Source: three-view drawing plus pictorial views. Frame: mm from the lowest corner of the part. A direction names the side the tool comes from. Coordinates: 2 decimals unless noted, no trailing zeros. Order: outer loops, then holes, each group sorted by start corner. A loop starts at its lowest first (then second) coordinate and runs counter-clockwise, first axis right, second up. Notation, with made-up numbers: (-13.75, -31.5) - (4.25, -31.5) arc R27 cw to (4.25, -8.5) - close; hole circle Ø9 at (-39, 49). An arc over 180 degrees is marked (long way). One line per question, with ' | ' between items.
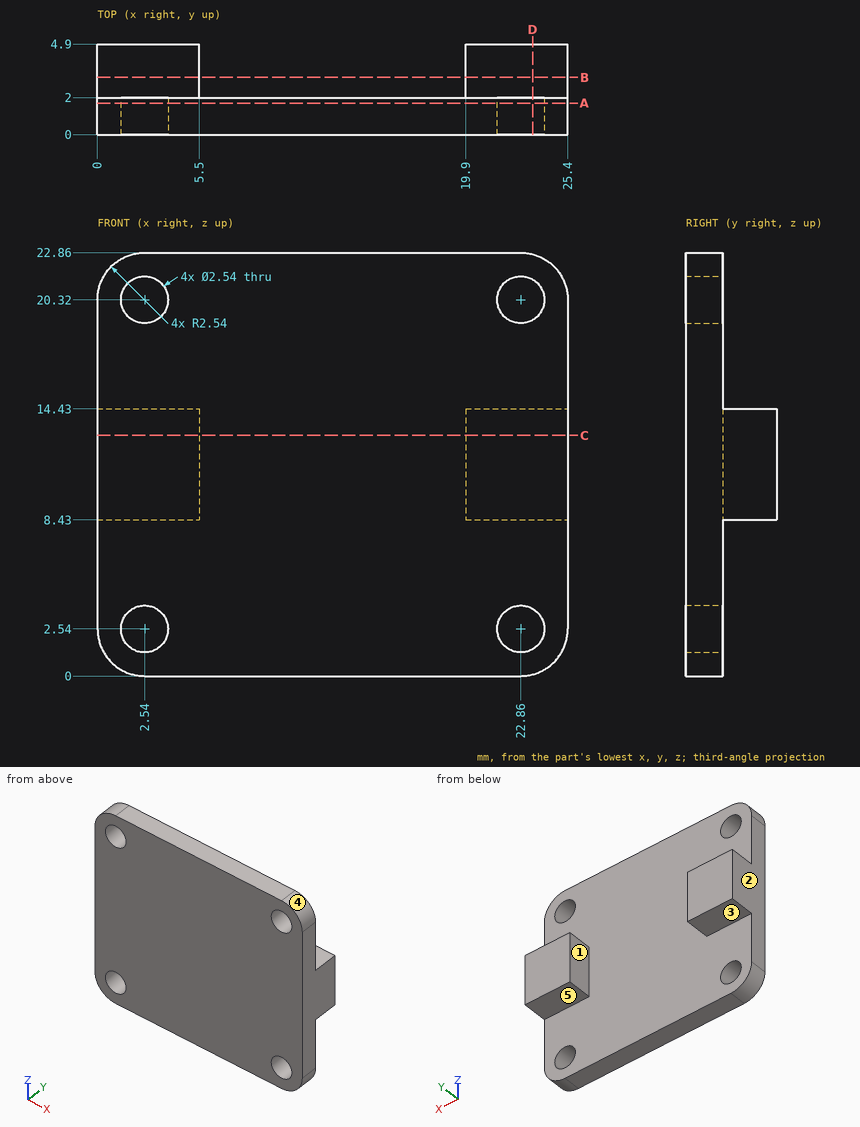
(1) Pin query (flat end, axial travel): P1, Ø10, axis at x = 7, z = 5.5, coming from the +Y side; P2, Ø3, axis at x = 2.54, z = 20.32, coming from the +Y side; P3, Ø1.5, axis at x = 23, y = 3.5, coming from the -Z side; P4, Ø1, axis at x = 13, y = 4, coming from the -Z side. Return the tip coordinate at first contact, or that it passes through.
Taken from the geometry:
P1: stops at y = 4.9 | P2: stops at y = 2 | P3: stops at z = 8.43 | P4: passes through
(2) Pull-direction query (X, two-part tool) for the marked faces 1, 2 and 3; classes: pulls with the +X half, pulls with the -X half, needs draft (parallel to the pull), parting line crosses it, or undercut.
Taken from the geometry:
face 1: undercut | face 2: pulls with the -X half | face 3: needs draft
(3) Cut plane C-C (z = 13). Return the cut outline in (x, y), and give its area (3 significant figures).
Taken from the geometry:
outline: (0, 0) - (25.4, 0) - (25.4, 4.9) - (19.9, 4.9) - (19.9, 2) - (5.5, 2) - (5.5, 4.9) - (0, 4.9) - close | area: 82.7 mm²
(4) Material intervals for L1, parallel to X at y = 1.05, z = 2.54; L2, parallel to Z at x = 2.54, y = 1.25; L3, parallel to Z at x = 1.75, y = 1.9, sorted ascending. Write a range as from..to.
Taken from the geometry:
L1: x = 0..1.27, 3.81..21.59, 24.13..25.4 | L2: z = 0..1.27, 3.81..19.05, 21.59..22.86 | L3: z = 0.13..1.55, 3.53..19.33, 21.31..22.73
(5) Cut plane A-A (y = 1.7). Return the cut outline in (x, z).
Taken from the geometry:
outline: (0, 2.54) arc R2.54 ccw to (2.54, 0) - (22.86, 0) arc R2.54 ccw to (25.4, 2.54) - (25.4, 20.32) arc R2.54 ccw to (22.86, 22.86) - (2.54, 22.86) arc R2.54 ccw to (0, 20.32) - close; hole circle Ø2.54 at (2.54, 2.54); hole circle Ø2.54 at (2.54, 20.32); hole circle Ø2.54 at (22.86, 2.54); hole circle Ø2.54 at (22.86, 20.32)
(6) Cut plane B-B (y = 3.1). Return the cut outline in (x, z).
Taken from the geometry:
outline: (0, 8.43) - (5.5, 8.43) - (5.5, 14.43) - (0, 14.43) - close; (19.9, 8.43) - (25.4, 8.43) - (25.4, 14.43) - (19.9, 14.43) - close
(7) Cut plane D-D (x = 23.5). Return the cut outline in (y, z), and give its area (3 significant figures).
Taken from the geometry:
outline: (0, 0.08) - (2, 0.08) - (2, 1.44) - (0, 1.44) - close; (0, 3.64) - (2, 3.64) - (2, 8.43) - (4.9, 8.43) - (4.9, 14.43) - (2, 14.43) - (2, 19.22) - (0, 19.22) - close; (0, 21.42) - (2, 21.42) - (2, 22.78) - (0, 22.78) - close | area: 54.0 mm²
(8) Set-up query: the marked faces 4 and 5. Return all of +Z, -Z, +X, -X, +Y, -Y with unobstructed straight access to the full face (end or side cutting, diameter ignored); none if empty.
Taken from the geometry:
face 4: +Z, +X, +Y, -Y | face 5: -Z, +X, -X, +Y
